Build history of the part. All positions in model axes, mm. A direction names the side the tool comes from. Round coordinates to 2 decimals unless told otherwise and drop trailing zeros. Write each loop counter-clockwise with the first axis right and the second up, starting at its lowest first coordinate (ties: lowest second). Pieces come first, ordered by that corner, then holes. Notation, with made-up numbers: (-7.5, 48.5) -> (12.5, 48.5) arc R33 cw to (12.5, 84.5) -> close; hole circle Ø11 at (21, 52). An arc over 180 degrees is marked (long way). Return JSON: item names as keys, results as strings.
from build123d import *

# Parameters (mm, degrees)
BOSS_EXTRUDE2_DEPTH         = 12.7
CUT_EXTRUDE1_DEPTH          = 7.62
SKETCH3_R                   = 3.3
CUT_EXTRUDE3_DEPTH          = 5.08
FILLET1_SIZE                = 2.54
F_1_4_CLEARANCE_HOLE1_D     = 6.7564
SKETCH8_R                   = 5.08
CUT_EXTRUDE4_DEPTH          = 125.929525349
CUT_EXTRUDE5_DEPTH          = 129.230913422
BOSS_EXTRUDE3_DEPTH         = 25.4
F_1_4_CLEARANCE_HOLE2_D     = 6.7564
F_1_4_CLEARANCE_HOLE2_DEPTH = 12.7
F_1_4_CLEARANCE_HOLE2_TIP   = 2.029827343
SKETCH14_R                  = 5.08
CUT_EXTRUDE6_DEPTH          = 6.604
CHAMFER1_SIZE               = 2.54


with BuildPart() as part:
    # Sketch1 → Boss-Extrude2 (new, symmetric)
    with BuildSketch(Plane.XY):
        Polygon((-121.836586579, 6.35), (-121.836586579, 0), (0, 0), (-115.262582833, 30.884515988), align=None)
    extrude(amount=BOSS_EXTRUDE2_DEPTH, both=True)

    # Sketch2 → Cut-Extrude1 (cut, symmetric)
    with BuildSketch(Plane.XY):
        Polygon((-112.78857866, 20.490012472), (-112.245058665, 22.518456707), (-106.256318542, 20.913778627), (-109.051564229, 10.481779703), (-115.040304352, 12.086457783), (-114.496784358, 14.114902018), align=None)
        Polygon((-79.832423525, 21.391033413), (-110.355679636, 29.569715239), (-112.245058665, 22.518456707), (-106.256318542, 20.913778627), (-109.051564229, 10.481779703), (-84.517048242, 3.907775958), align=None)
    extrude(amount=CUT_EXTRUDE1_DEPTH, both=True, mode=Mode.SUBTRACT)

    # Sketch3 → Cut-Extrude3 (cut)
    with BuildSketch(Plane(origin=(-115.262582833, 30.884515988, 0), x_dir=(0, 0, 1), z_dir=(-0.96592582628907, 0.25881904510251447, 0))):
        with Locations(Location((0, -12.7, 0), (0, 0, 270))):
            Circle(SKETCH3_R)
    extrude(amount=-CUT_EXTRUDE3_DEPTH, mode=Mode.SUBTRACT)

    # Fillet1
    # a fillet whose section is not a circle: 2.54 mm, written as the material it adds along each edge
    with BuildSketch(Plane(origin=(-84.517048242, 3.907775958, 7.62), x_dir=(0.25881904510251297, 0.9659258262890703, 0), z_dir=(0, 0, -1))) as fillet1_piece_1:
        with BuildLine():
            add(Edge.make_bspline([(FILLET1_SIZE, 0), (FILLET1_SIZE * 0.831801948466, 0), (FILLET1_SIZE * 0.663603896932, 0), (FILLET1_SIZE * 0.292893218813, -FILLET1_SIZE * 0.0716919198361), (FILLET1_SIZE * 0.0716919198361, -FILLET1_SIZE * 0.292893218813), (0, -FILLET1_SIZE * 0.663603896932), (0, -FILLET1_SIZE * 0.831801948466), (0, -FILLET1_SIZE)], knots=[0, 0, 0, 0, 0, 0, 0.5, 0.5, 1, 1, 1, 1, 1, 1], degree=5))
            Line((0, -FILLET1_SIZE), (0, 0))
            Line((0, 0), (FILLET1_SIZE, 0))
        make_face()
    extrude(amount=15.24)
    with BuildSketch(Plane(origin=(-115.040304352, 12.086457783, 7.62), x_dir=(0.25881904510251585, 0.9659258262890695, 0), z_dir=(0.9659258262890696, -0.2588190451025158, 0))) as fillet1_piece_2:
        with BuildLine():
            add(Edge.make_bspline([(FILLET1_SIZE, 0), (FILLET1_SIZE * 0.831801948466, 0), (FILLET1_SIZE * 0.663603896932, 0), (FILLET1_SIZE * 0.292893218813, -FILLET1_SIZE * 0.0716919198361), (FILLET1_SIZE * 0.0716919198361, -FILLET1_SIZE * 0.292893218813), (0, -FILLET1_SIZE * 0.663603896932), (0, -FILLET1_SIZE * 0.831801948466), (0, -FILLET1_SIZE)], knots=[0, 0, 0, 0, 0, 0, 0.5, 0.5, 1, 1, 1, 1, 1, 1], degree=5))
            Line((0, -FILLET1_SIZE), (0, 0))
            Line((0, 0), (FILLET1_SIZE, 0))
        make_face()
    extrude(amount=37.95)
    with BuildSketch(Plane(origin=(-115.040304352, 12.086457783, -7.62), x_dir=(0.25881904510251585, 0.9659258262890695, 0), z_dir=(0.9659258262890696, -0.2588190451025158, 0))) as fillet1_piece_3:
        with BuildLine():
            add(Edge.make_bspline([(FILLET1_SIZE, 0), (FILLET1_SIZE * 0.831801948466, 0), (FILLET1_SIZE * 0.663603896932, 0), (FILLET1_SIZE * 0.292893218813, FILLET1_SIZE * 0.0716919198361), (FILLET1_SIZE * 0.0716919198361, FILLET1_SIZE * 0.292893218813), (0, FILLET1_SIZE * 0.663603896932), (0, FILLET1_SIZE * 0.831801948466), (0, FILLET1_SIZE)], knots=[0, 0, 0, 0, 0, 0, 0.5, 0.5, 1, 1, 1, 1, 1, 1], degree=5))
            Line((0, FILLET1_SIZE), (0, 0))
            Line((0, 0), (FILLET1_SIZE, 0))
        make_face()
    extrude(amount=37.95)

    # 1/4 Clearance Hole1 (through all)
    with Locations(Plane(origin=(0, 0, 0), x_dir=(-1, 0, 0), z_dir=(0, -1, 0))):
        with Locations((71.036586579, 0)):
            Hole(F_1_4_CLEARANCE_HOLE1_D / 2)

    # Sketch8 → Cut-Extrude4 (cut, through all)
    with BuildSketch(Plane(origin=(0, 6.35, 0), x_dir=(-1, 0, 0), z_dir=(0, -1, 0))):
        with Locations(Location((71.036586579, 0, 0), (0, 0, 90))):
            Circle(SKETCH8_R)
    extrude(amount=-CUT_EXTRUDE4_DEPTH, mode=Mode.SUBTRACT)

    # Sketch9 → Cut-Extrude5 (cut, through all)
    with BuildSketch(Plane.XY.offset(12.7)):
        Polygon((-12.7, 3.402954744), (-12.7, 0), (0, 0), align=None)
    extrude(amount=-CUT_EXTRUDE5_DEPTH, mode=Mode.SUBTRACT)

    # Sketch10 → Boss-Extrude3 (add)
    with BuildSketch(Plane.XY.offset(12.7)):
        Polygon((-12.7, 3.402954744), (-12.7, 41.502954744), (-25.4, 41.502954744), (-25.4, 6.805909488), align=None)
    extrude(amount=-BOSS_EXTRUDE3_DEPTH)

    # 1/4 Clearance Hole2
    with Locations(Plane(origin=(-12.7, 0, 0), x_dir=(0, 0, -1), z_dir=(1, 0, 0))):
        with Locations((0, 28.802954744)):
            Hole(F_1_4_CLEARANCE_HOLE2_D / 2, depth=F_1_4_CLEARANCE_HOLE2_DEPTH)
            with Locations((0, 0, -(F_1_4_CLEARANCE_HOLE2_DEPTH + F_1_4_CLEARANCE_HOLE2_TIP / 2))):  # 118° drill point
                Cone(0, F_1_4_CLEARANCE_HOLE2_D / 2, F_1_4_CLEARANCE_HOLE2_TIP, mode=Mode.SUBTRACT)

    # Sketch14 → Cut-Extrude6 (cut)
    with BuildSketch(Plane.ZY.offset(25.4)):
        with Locations(Location((0, 28.802954744, 0), (0, 0, 270))):
            Circle(SKETCH14_R)
    extrude(amount=-CUT_EXTRUDE6_DEPTH, mode=Mode.SUBTRACT)

    # Chamfer1
    chamfer1_edges = [part.edges().sort_by_distance(p)[0] for p in [
        (-25.4, 41.502954744, 0),
    ]]
    chamfer(chamfer1_edges, length=CHAMFER1_SIZE)

    # Fillet2
    # a fillet whose section is not a circle: 5.08 mm, written as the material it adds along each edge (its section moved 0.00015 mm through the faces so that the kernel can cut it)
    with BuildSketch(Plane(origin=(-25.4, 6.805909488, 12.7), x_dir=(2.2657292946534733e-05, 0.9999999997433235, 0), z_dir=(0, 0, -1))) as fillet2_piece_1:
        with BuildLine():
            add(Edge.make_bspline([(6.620384896, 0), (5.560159502, 2.4022e-05), (4.499934108, 4.8044e-05), (2.201778974, -0.538520049), (1.089942696, -1.987425322), (1.164425276, -4.346667776), (1.438808597, -5.370773083), (1.713191917, -6.39487839)], knots=[0, 0, 0, 0, 0, 0, 0.5, 0.5, 1, 1, 1, 1, 1, 1], degree=5))
            Line((1.713191917, -6.39487839), (1.615053258, -6.421172181))
            ThreePointArc((1.615053258, -6.421172181), (0.758529744, -3.223713577), (-0.09813866, -0.026293791))
            Line((-0.09813866, -0.026293791), (2.302e-06, 0.1016))
            ThreePointArc((2.302e-06, 0.1016), (3.310194748, 0.101525), (6.620387198, 0.1016))
            Line((6.620387198, 0.1016), (6.620384896, 0))
        make_face()
    extrude(amount=25.4)


solid = part.part
Q1. Saw through at A-A on y = 27. List the corners of the cut face in (x, z), then the cut area to 3 significant figures.
Verdict:
{"outline": "(-116.3, -12.7) -> (-100.77, -12.7) -> (-100.77, -7.62) -> (-111.04, -7.62) -> (-111.04, 7.62) -> (-100.77, 7.62) -> (-100.77, 12.7) -> (-116.3, 12.7) -> close; (-25.4, -12.7) -> (-12.7, -12.7) -> (-12.7, -2.86) -> (-18.8, -2.86) -> (-18.8, -4.75) -> (-25.4, -4.75) -> close; (-25.4, 4.75) -> (-18.8, 4.75) -> (-18.8, 2.86) -> (-12.7, 2.86) -> (-12.7, 12.7) -> (-25.4, 12.7) -> close", "area": "463 mm²"}
Q2. Pin check, flat tips, straight feed: pin 1 Ø8 at (x, z) = (-81.5, 0.5) entering from -Y; pin 2 Ø5 at (x, z) = (-48, -2.5) entering from +Y; pin 3 Ø5 at (y, z) = (31, -2) entering from -X; pin 4 Ø8 at (x, z) = (-73.5, -2.5) entering from +Y. Stop position of each tip, or through.
Verdict:
{"pin 1": "stops at y = 0", "pin 2": "stops at y = 13.53", "pin 3": "stops at x = -115.9", "pin 4": "stops at y = 20.77"}
Q3. 3-axis set-ups, long thin cutter, end or side, ignore diameter. For faces 1 (the flat face through (-121.837, 3, 0)), 2 (the flat face through (-63.55, 17.03, 0.18)), 3 (the cylindrical face through (-15.8, 25.5, -0.7)), 4 (the cylindrical face through (-75.996, 13.274, 1.101)), 5 (the cylindrical face through (-22.14, 33.88, 0.22)): which of +Z, -Z, +X, -X, +Y, -Y reach the whole face in a straight line?
Verdict:
{"face 1": "+Z, -Z, -X, +Y, -Y", "face 2": "+Z, -Z, +Y", "face 3": "+X", "face 4": "+Y", "face 5": "none"}
Q4. Saw through at B-B on x = -24. List the corners of the cut face in (y, z).
Verdict:
{"outline": "(0, -12.7) -> (40.36, -12.7) -> (40.36, 12.7) -> (0, 12.7) -> close; hole circle Ø10.16 at (28.8, 0)"}
Q5. Saw through at C-C on x = -35.5. List the corners of the cut face in (y, z), then the cut area to 3 significant figures.
Verdict:
{"outline": "(0, -12.7) -> (9.51, -12.7) -> (9.51, 12.7) -> (0, 12.7) -> close", "area": "242 mm²"}
Q6. Wall check: L1, parallel to Y at x = -14.25, z = 0; L2, parallel to Z at x = -103.5, y = 23; L3, parallel to X at y = 24.5, z = -2.75. Give the ranges that are in metal, low to high.
Verdict:
{"L1": "y = 0 to 25.42, 32.18 to 41.5", "L2": "z = -12.7 to -7.62, 7.62 to 12.7", "L3": "x = -116.97 to -111.71, -25.4 to -12.7"}
Q7. Two-plate mould, pull along Y, no slides. Class faces 6 (the flat face through (-12.7, 20, 0)), 7 (the flat face through (-24.148, 40.215, 0.178)), 8 (the flat face through (-18.796, 25, -1)), 9 (the flat face through (-68, 0, 3)): +Y half, -Y half, draft (parallel to the pull), parting line (faces both ways), or undercut.
Verdict:
{"face 6": "draft", "face 7": "+Y half", "face 8": "undercut", "face 9": "-Y half"}
